Autodesk Inventor part; units mm, degrees
ref_plane "YZ Plane" through (0, 0, 0) normal (1, 0, 0) x (0, 1, 0)
ref_plane "XZ Plane" through (0, 0, 0) normal (0, 1, 0) x (-1, 0, 0)
ref_plane "XY Plane" through (0, 0, 0) normal (0, 0, 1) x (1, 0, 0)
sketch "Sketch1" plane through (0, 0, 0) normal (0, 1, 0) x (-1, 0, 0)
  line L0 (7.5, 7.75) -> (-7.5, 7.75)
  line L1 (-7.5, 7.75) -> (-7.5, -7.75)
  line L2 (-7.5, -7.75) -> (7.5, -7.75)
  line L3 (7.5, -7.75) -> (7.5, 7.75)
  line L4 (7.5, 7.75) -> (-7.5, -7.75) construction
  line L5 (-7.5, 7.75) -> (7.5, -7.75) construction
  point P0 (0, 0)
  dimension "d0" = 15
  dimension "d1" = 15.5
extrude "Extrusion1" add sketch "Sketch1" along normal blind 6
sketch "Sketch2" plane through (0, 6, 0) normal (0, 1, 0) x (1, 0, 0)
  line L0 (7.5, -7.75) -> (7.5, 7.75)
  line L1 (-7.5, 7.75) -> (-7.5, -7.75)
  line L2 (-7.5, 4.275) -> (-2.4, 4.275)
  line L3 (-2.4, 4.275) -> (-2.4, -4.275)
  line L4 (-2.4, -4.275) -> (-7.5, -4.275)
  line L5 (-7.5, 0) -> (-2.4, -4.275) construction
  line L6 (-2.4, 4.275) -> (-7.5, 0) construction
  line L7 (-7.5, 4.275) -> (-7.5, -4.275)
  point P0 (0, 0)
  point P1 (-7.5, 0)
  dimension "d4" = 15
  dimension "d5" = 5.1
  dimension "d6" = 8.55
extrude "Extrusion2" cut sketch "Sketch2" against normal blind 8.25
sketch "Sketch3" plane through (-2.4, 6, -4.275) normal (-1, 0, 0) x (0, 0, 1)
  line L0 (0, -1) -> (8.55, -1)
  line L1 (8.55, -1) -> (8.55, -6)
  line L2 (0, -6) -> (0, -1)
  line L3 (0, -1) -> (4.275, -6) construction
  line L4 (8.55, -1) -> (4.275, -6) construction
  line L5 (0, -6) -> (8.55, -6)
  dimension "d9" = 5
extrude "Extrusion3" cut sketch "Sketch3" against normal blind 2
properties part number "TAPA3_3DPrint"
For this review, take the finished solid that the model builds, in its own axes (mm). A direction names the side the tool comes from. Give positions to 0.01 mm unless a question says otherwise; leave off trailing zeros. Write each loop counter-clockwise with the first axis right and the second up, starting at its lowest first coordinate (ties: lowest second). Pieces come first, ordered by that corner, then holes. Notation, with made-up numbers: M -33,42.5 L 24,42.5 A36 ccw 24,77.5 Z; hole C 13.5,48.25 d2. An arc over 180 degrees is marked long. Answer as CSV lines item,"result".
1. Consider section A-A, the plane y = 4.6. Write out the cut boundary in (x, z) (3 decimals).
Findings:
outline,"M -7.5,-7.75 L 7.5,-7.75 L 7.5,7.75 L -7.5,7.75 L -7.5,4.275 L -0.4,4.275 L -0.4,-4.275 L -7.5,-4.275 Z"
2. Wall thickness on line 1 (Z direction, x = -6, y = 0.9) (3 decimals); line 2 (X direction, y = 2.3, z = -1); line 3 (X direction, y = 5.4, z = 2.5): over which ranges is each line inside the solid? List them lowest first.
Findings:
line 1,"z = -7.75 to -4.275, 4.275 to 7.75"
line 2,"x = -0.4 to 7.5"
line 3,"x = -2.4 to 7.5"
3. Consider section C-C, the plane z = 0.5. Write out the cut boundary in (x, y), then the cut area to 3 significant figures.
Findings:
outline,"M -2.4,5 L -0.4,5 L -0.4,0 L 7.5,0 L 7.5,6 L -2.4,6 Z"
area,"49.4 mm2"
4. For pin 1 (1.5 mm diameter, centred on y = 1.5, z = 1, fed in from -X); pin 2 (1.6 mm diameter, centred on x = -1.5, z = 0, fed in from -Y); pin 3 (0.8 mm diameter, centred on y = 5.5, z = -1.5, fed in from -X), all flat-tipped, find the tip position at first contact; note any pin that passes through.
Findings:
pin 1,"stops at x = -0.4"
pin 2,"stops at y = 5"
pin 3,"stops at x = -2.4"
5. Draft analysis for pull direction Z (two halves, no side actions). For faces 4 (the flat face through (-0.4, 3, 0)), 5 (the flat face through (0, 3, -7.75)), 6 (the flat face through (-7.5, 3, -6)), state which applies: +Z half, -Z half, draft (parallel to the pull), parting line (faces both ways), or undercut.
Findings:
face 4,"undercut"
face 5,"-Z half"
face 6,"draft"
6. For faces 1 (the flat face through (0, 3, 7.75)), 2 (the flat face through (-2.4, 5.5, -0.1)), 3 (the flat face through (-1, 5, 0)), list the 3-axis set-ups (+Z, -Z, +X, -X, +Y, -Y) from which the entire face can be reached by the end or side of a thin tool; tool diameter is ignored.
Findings:
face 1,"+Z, +X, -X, +Y, -Y"
face 2,"-X, +Y, -Y"
face 3,"-X, -Y"
7. Consider section B-B, the plane x = -6.5. Write out the cut boundary in (y, z) (3 decimals).
Findings:
outline,"M 0,-7.75 L 6,-7.75 L 6,-4.275 L 0,-4.275 Z; M 0,4.275 L 6,4.275 L 6,7.75 L 0,7.75 Z"
